Could you check a few things on this model? Use its own coordinates, in mm. Give positions to 0.01 mm unless a question says otherwise; leave off trailing zeros. Loops run counter-clockwise (first coordinate to the right, second up) from the corner with the lowest first, then second, coordinate; pieces in that order, holes last. Notation, with made-up numbers: M -40,33.25 L 19,33.25 A30 cw 19,66.25 Z; hole C -16,5.25 d4. An arc over 180 degrees is marked long. Answer in a Markdown table with one row per item. Add a question column.
```python
from build123d import *

# Parameters (mm, degrees)
TAP_DRILL_FOR_M4X0_7_TAP2_D     = 3.3
TAP_DRILL_FOR_M4X0_7_TAP2_DEPTH = 6
TAP_DRILL_FOR_M4X0_7_TAP2_TIP   = 0.991420021


with BuildPart() as part:
    # Sketch2 → Revolve1 (revolve)
    with BuildSketch(Plane.XY):
        with BuildLine():
            Line((-7.5, 0), (7.5, 0))
            ThreePointArc((7.5, 0), (0, 7.5), (-7.5, 0))
        make_face()
    revolve(axis=Axis((-7.5, 0, 0), (1, 0, 0)))

    # Tap Drill for M4x0.7 Tap2
    with Locations(Plane(origin=(0, 7.5, 0), x_dir=(1, 0, 0), z_dir=(0, 1, 0))):
        with Locations((0, 0)):
            Hole(TAP_DRILL_FOR_M4X0_7_TAP2_D / 2, depth=TAP_DRILL_FOR_M4X0_7_TAP2_DEPTH)
            with Locations((0, 0, -(TAP_DRILL_FOR_M4X0_7_TAP2_DEPTH + TAP_DRILL_FOR_M4X0_7_TAP2_TIP / 2))):  # 118° drill point
                Cone(0, TAP_DRILL_FOR_M4X0_7_TAP2_D / 2, TAP_DRILL_FOR_M4X0_7_TAP2_TIP, mode=Mode.SUBTRACT)

    # Chamfer1
    # the kernel refuses this chamfer: 0.25, 0.209117546 mm, written as the material it takes off along each edge
    with BuildSketch(Plane(origin=(-1e-09, 7.316249039, -3e-09), x_dir=(-1.0, 0, 1.5237922439259502e-09), z_dir=(1.5237922439259502e-09, 0, 1.0))) as chamfer1_piece_1:
        with BuildLine():
            Line((1.851597136, 0.048402863), (1.649999997, 0.250000002))
            Line((1.649999997, 0.250000002), (1.649999999, 0))
            ThreePointArc((1.649999999, 0), (1.75350475, 0.024114846), (1.851597136, 0.048402863))
        make_face()
    revolve(axis=Axis((-1e-09, 7.316249039, -3e-09), (0, -1, 0)), revolution_arc=180.000000175, mode=Mode.SUBTRACT)
    with BuildSketch(Plane(origin=(0, 7.316249039, 3e-09), x_dir=(1.0, 0, -1.755349969310666e-09), z_dir=(-1.755349969310666e-09, 0, -1.0))) as chamfer1_piece_2:
        with BuildLine():
            Line((1.851597137, 0.048402863), (1.649999997, 0.250000003))
            Line((1.649999997, 0.250000003), (1.65, 0))
            ThreePointArc((1.65, 0), (1.75350475, 0.024114847), (1.851597137, 0.048402863))
        make_face()
    revolve(axis=Axis((0, 7.316249039, 3e-09), (0, -1, 0)), revolution_arc=180.000000201, mode=Mode.SUBTRACT)


solid = part.part
```
Item 1: Suppose I cut it at A-A (x = -6). List the corners of the cut face in (y, z) for me, then the cut area to 3 significant figures.
Item 2: I need wall thicknesses on L1, parallel to Z at x = 0, y = 5.95; L2, parallel to Z at x = 1.25, y = 6.5; L3, parallel to X at y = 5.45, z = 0. Which ranges of each line are inside material? Lowest first, please.
Item 3: For P1, Ø1.5, axis at y = 5, z = -0.5, coming from the +X side; P2, Ø5, axis at x = -3.5, y = -4.5, coming from the +Z side; P3, Ø5, axis at x = 1, z = -1.5, coming from the +Y side; P4, Ø5, axis at x = 4, z = 5, coming from the +Y side, each with a flat end and sliding along its axis, tell me the tip position at first contact or that it passes through.
Item 4: Suppose I cut it at C-C (y = 3.25). List the corners of the cut face in (x, z) for me, then the cut area to 3 significant figures.
Item 5: Suppose I cut it at B-B (y = -5.25). List the corners of the cut face in (x, z) for me.
Values found:
| question | item | result |
|---|---|---|
| 1 | outline | C 0,0 d9 |
| 1 | area | 63.6 mm² |
| 2 | L1 | -4.57 to -1.65, 1.65 to 4.57 |
| 2 | L2 | -3.53 to -1.08, 1.08 to 3.53 |
| 2 | L3 | -5.15 to -1.65, 1.65 to 5.15 |
| 3 | P1 | x = 6.16 |
| 3 | P2 | z = 6.78 |
| 3 | P3 | y = 7.27 |
| 3 | P4 | y = 6.4 |
| 4 | outline | C 0,0 d13.52; hole C 0,0 d3.3 |
| 4 | area | 135 mm² |
| 5 | outline | C 0,0 d10.71 |
